```python
from build123d import *

# Parameters (mm, degrees)
SKETCH1_R           = 3.911052803
BOSS_EXTRUDE1_DEPTH = 4
CAVITY1_OUTLINE_W   = 12.415
CAVITY1_OUTLINE_H   = 5.700748897


# Read off the part's stored shape, not the designer's step: Cavity1
with BuildPart() as part:
    # Sketch1 → Boss-Extrude1 (new body)
    with BuildSketch(Plane(origin=(0, 0, 0), x_dir=(1, 0, 0), z_dir=(0, 1, 0))):
        with BuildLine():
            Line((0, 0), (30, 0))
            Line((30, 0), (25.709430043, 75.411524479))
            ThreePointArc((25.709430043, 75.411524479), (22.592877256, 82.112613927), (15.725576294, 84.84348898))
            Line((15.725576294, 84.84348898), (15.172794511, 84.84348898))
            Line((15.172794511, 84.84348898), (14.566572295, 84.84348898))
            ThreePointArc((14.566572295, 84.84348898), (7.713312448, 82.125853257), (4.584985356, 75.450054873))
            Line((4.584985356, 75.450054873), (0, 0))
        make_face()
        with Locations(Location((15.172794511, 74.362549593, 0), (0, 0, 270))):
            Circle(SKETCH1_R, mode=Mode.SUBTRACT)
    extrude(amount=BOSS_EXTRUDE1_DEPTH)

    # Cavity1 outline → Cavity1 (revolve, cut)
    with BuildSketch(Plane(origin=(19.189357323, 5.518997389, 9.104198025), x_dir=(0.9996334354377989, 0.02380958372693479, -0.012887919831146358), z_dir=(0, -0.47602788353146924, -0.8794301871669804))):
        with Locations((6.2075, -2.156922497)):
            Rectangle(CAVITY1_OUTLINE_W, CAVITY1_OUTLINE_H)
    revolve(axis=Axis((19.189357323, 5.518997389, 9.104198025), (0.027073875873690006, -0.8791078192254351, 0.47585338857874704)), mode=Mode.SUBTRACT)


solid = part.part
```
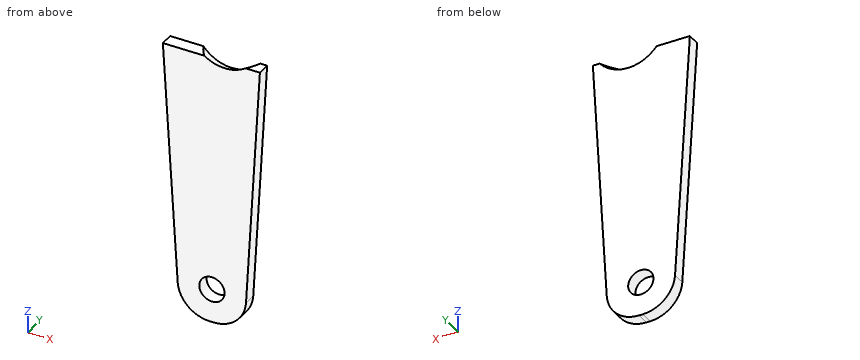
Source: CAD feature listing. Evaluate the final solid. Frame: model axes, mm. Give positions to 0.01 mm unless a question says otherwise; leave off trailing zeros. Write each loop counter-clockwise with the first axis right and the second up, starting at its lowest first coordinate (ties: lowest second). Pieces come first, ordered by that corner, then holes. Notation, with made-up numbers: (-26, 51) - (10, 51) arc R13 ccw to (10, 63) - close; hole circle Ø8 at (-15, 13.5). An arc over 180 degrees is marked (long way). One line per item, written item: value. Start each with the question number.
Q1. Section query C-C, the plane x = 7.75. Return the cut outline in (y, z).
Q2. Section query B-B, the plane z = -48. Return the cut outline in (x, y), then the cut area to 3 significant figures.
Q3. Material intervals for probe 1 along Z at (x, y) = (15.25, 1.1); probe 2 along Z at (x, y) = (14, 1.2); probe 3 along Z at (x, y) = (8.5, 1.45), sorted ascending. Write a range as from..to.
Q4. First-contact query: pin 1 Ø1.5 at (x, y) = (19.5, 3) entering from +Z; pin 2 Ø1 at (y, z) = (1, -10.5) entering from +X; pin 3 Ø2 at (x, y) = (23.5, 2.5) entering from +Z. Flat tips, straight axial feed; report the tip coordinate or a pass-through.
Q5. Section query A-A, the plane z = -71.5. Return the cut outline in (x, y), then the cut area to 3 significant figures.
Answer:
1. outline: (0, -82.16) - (4, -82.16) - (4, 0) - (0, 0) - close
2. outline: (2.92, 0) - (27.27, 0) - (27.27, 4) - (2.92, 4) - close
2. area: 97.4 mm2
3. probe 1: z = -84.84..-78.27, -70.45..-1.91
3. probe 2: z = -84.83..-78.09, -70.63..-1.4
3. probe 3: z = -82.79..0
4. pin 1: stops at z = -3.24
4. pin 2: stops at x = 29.43
4. pin 3: stops at z = -1.77
5. outline: (4.34, 0) - (12.51, 0) - (12.51, 4) - (4.34, 4) - close; (17.84, 0) - (25.93, 0) - (25.93, 4) - (17.84, 4) - close
5. area: 65.0 mm2
